Build history of the part. All positions in model axes, mm. A direction names the side the tool comes from. Coordinates: 2 decimals unless noted, no trailing zeros. Loops run counter-clockwise (first coordinate to the right, second up) from the corner with the lowest first, then second, coordinate; pieces in that order, holes last. Notation, with made-up numbers: (17, 13) -> (57, 13) arc R26 ccw to (57, 48) -> close; hole circle Ø10 at (-12.75, 34). An arc over 180 degrees is marked (long way). One line per item, written item: value. Start each with the question number.
Solid Edge part; units mm, degrees
sketch "Sketch1" plane through (0, 0, 0) normal (0, 0, 1) x (1, 0, 0)
  line L0 (-35, -25) -> (35, -25)
  line L1 (35, -25) -> (35, 25)
  line L2 (35, 25) -> (-35, 25)
  line L3 (-35, 25) -> (-35, -25)
  dimension "D1" = 35
  dimension "D2" = 35
extrude "Protrusion1" add sketch "Sketch1" along normal blind 20
fillet "Round1" radius 10 4 edges at (-35, -25, 10) (-35, 25, 10) (35, -25, 10) (35, 25, 10)
hole "Hole1" at (-22.5, 0, 20) direction (0, 0, -1) diameter 12 end up to next
hole "Hole2" at (22.5, 0, 20) direction (0, 0, -1) diameter 12 end up to next
sketch "Sketch2" plane through (0, 0, 0) normal (1, 0, 0) x (0, 1, 0)
  line L0 (-10, 20) -> (10, 20)
  line L1 (10, 20) -> (10, 50)
  line L2 (10, 50) -> (-10, 50)
  line L3 (-10, 50) -> (-10, 20)
  dimension "D1" = 10
  dimension "D2" = 10
extrude "Protrusion2" add sketch "Sketch2" along normal mid plane 10
fillet "Round2" radius 10 2 edges at (0, -10, 50) (0, 10, 50)
properties material "알루미늄, 1060"
Item 1: Band-saw the part on D-D, the plane z = 26.5. List the corners of the cut face in (x, y).
Item 2: Band-saw the part on C-C, the plane y = 3.5. List the corners of the cut face in (x, z).
Item 3: Probe probe 1 along X at (y, z) = (0, 9); probe 2 along Y at (x, z) = (22.5, 7.25); probe 3 along X at (y, z) = (-9, 31). List the from-to ranges inside material, lowest first.
Item 4: Two-plate mould, pull along X, no slides. Class faces 5 (the face through (-28.357, 1.301, 10.14)), 6 (the face through (-31.99, 22.15, 10.14)), 7 (the face through (5, 0, 35)): +X half, -X half, draft (parallel to the pull), parting line (faces both ways), or undercut.
Item 5: Drop flat-ended pins along their axis: pin 1 Ø10 at (y, z) = (0.5, 34) entering from +X; pin 2 Ø14 at (x, y) = (22.5, 0) entering from +Z; pin 3 Ø19 at (x, y) = (-22.5, 0) entering from -Z; pin 4 Ø5 at (x, z) = (-1, 26) entering from +Y. Give the stop position or say it passes through.
Item 6: Band-saw the part on A-A, the plane x = -22.5. List the corners of the cut face in (y, z).
Item 7: Tool access for faces 1 (the face through (-5, 0, 35)), 2 (the face through (0, -10, 30)), 3 (the face through (0, 0, 0)), 4 (the face through (0, 10, 30)): list every direction of +Z, -Z, +X, -X, +Y, -Y with a clear straight run to the whole face (end or side of a thin tool).
Item 8: Band-saw the part on B-B, the plane z = 19. List the corners of the cut face in (x, y).
Worked out:
1. outline: (-5, -10) -> (5, -10) -> (5, 10) -> (-5, 10) -> close
2. outline: (-35, 0) -> (-27.37, 0) -> (-27.37, 20) -> (-35, 20) -> close; (-17.63, 0) -> (17.63, 0) -> (17.63, 20) -> (5, 20) -> (5, 49.37) -> (-5, 49.37) -> (-5, 20) -> (-17.63, 20) -> close; (27.37, 0) -> (35, 0) -> (35, 20) -> (27.37, 20) -> close
3. probe 1: x = -35 to -28.5, -16.5 to 16.5, 28.5 to 35
3. probe 2: y = -25 to -6, 6 to 25
3. probe 3: x = -5 to 5
4. face 5: undercut
4. face 6: -X half
4. face 7: +X half
5. pin 1: stops at x = 5
5. pin 2: stops at z = 20
5. pin 3: stops at z = 0
5. pin 4: stops at y = 10
6. outline: (-25, 0) -> (-6, 0) -> (-6, 20) -> (-25, 20) -> close; (6, 0) -> (25, 0) -> (25, 20) -> (6, 20) -> close
7. face 1: +Z, -X, +Y, -Y
7. face 2: +Z, +X, -X, -Y
7. face 3: -Z, +X, -X, +Y, -Y
7. face 4: +Z, +X, -X, +Y
8. outline: (-35, -15) arc R10 ccw to (-25, -25) -> (25, -25) arc R10 ccw to (35, -15) -> (35, 15) arc R10 ccw to (25, 25) -> (-25, 25) arc R10 ccw to (-35, 15) -> close; hole circle Ø12 at (-22.5, 0); hole circle Ø12 at (22.5, 0)
